Can you work these out from the model? Positions are in its coordinate system, mm. A direction names the side the tool comes from. Give positions to 0.01 mm unless a question says otherwise; leave off trailing zeros. Order: outer loops, then holes, each group sorted by start corner. A loop starts at its lowest first (then second) coordinate and runs counter-clockwise, first axis right, second up. Notation, with made-up numbers: M 27,58 L 85,58 A15 ccw 85,69 Z; hole C -7,86.5 d9. An arc over 180 degrees is marked long. Answer as a JSON object with one key per item and string values.
```python
from build123d import *

# Parameters (mm, degrees)
SKETCH2_W           = 2.25
SKETCH2_H           = 25
BOSS_EXTRUDE1_DEPTH = 4


with BuildPart() as part:
    # Sketch2 → Revolve1 (revolve)
    with BuildSketch(Plane.XY, mode=Mode.PRIVATE) as revolve1_sk:
        with Locations((1.125, 12.5)):
            Rectangle(SKETCH2_W, SKETCH2_H)
    revolve(revolve1_sk.sketch.rotate(Axis((0, 0, 0), (0, 1, 0)), 90), axis=Axis((0, 0, 0), (0, 1, 0)))

    # Sketch3 → Boss-Extrude1 (add)
    with BuildSketch(Plane(origin=(0, 25, 0), x_dir=(1, 0, 0), z_dir=(0, 1, 0))):
        Polygon((4.041451884, 0), (2.020725942, 3.5), (-2.020725942, 3.5), (-4.041451884, 0), (-2.020725942, -3.5), (2.020725942, -3.5), align=None)
    extrude(amount=BOSS_EXTRUDE1_DEPTH)


solid = part.part
```
1) I want a section at B-B on z = 1.75. Write out the boundary of the cut face in (x, y), and give its area (3 significant figures).
Results found:
{"outline": "M -3.03,25 L -1.41,25 L -1.41,0 L 1.41,0 L 1.41,25 L 3.03,25 L 3.03,29 L -3.03,29 Z", "area": "95.0 mm²"}
2) I'm going to push flat-ended pins straight in: pin 1 Ø2 at (x, y) = (-2, 12.5) entering from +Z; pin 2 Ø2 at (x, z) = (0, 0.5) entering from -Y. Where does each tip first touch, or does it pass through?
Results found:
{"pin 1": "stops at z = 2.02", "pin 2": "stops at y = 0"}
3) I need wall thicknesses on L1, parallel to Z at x = 1, y = 22; L2, parallel to Y at x = -2.5, z = 0.25. Which ranges of each line are inside material? Lowest first, please.
Results found:
{"L1": "z = -2.02 to 2.02", "L2": "y = 25 to 29"}
4) I want a section at C-C on y = 4.5. Write out the boundary of the cut face in (x, z).
Results found:
{"outline": "C 0,0 d4.5"}
5) I want a section at A-A on x = 0. Write out the boundary of the cut face in (y, z), and give its area (4 significant figures).
Results found:
{"outline": "M 0,-2.25 L 25,-2.25 L 25,-3.5 L 29,-3.5 L 29,3.5 L 25,3.5 L 25,2.25 L 0,2.25 Z", "area": "140.5 mm²"}
6) For faces 1 (the face through (2, 25, -2)), 2 (the face through (3.045, 26.972, -1.726)), which set-ups out of +Z, -Z, +X, -X, +Y, -Y let a thin tool reach every point of the face, with its end or its side?
Results found:
{"face 1": "-Y", "face 2": "-Z, +X, +Y, -Y"}
